Job drawing, mm, ordinate dimensions from the low corner. One solid piece. A direction names the side the tool comes from. Round coordinates to 2 decimals unless told otherwise and drop trailing zeros. Loops run counter-clockwise (first coordinate to the right, second up) from the corner with the lowest first, then second, coordinate; pieces in that order, holes last.
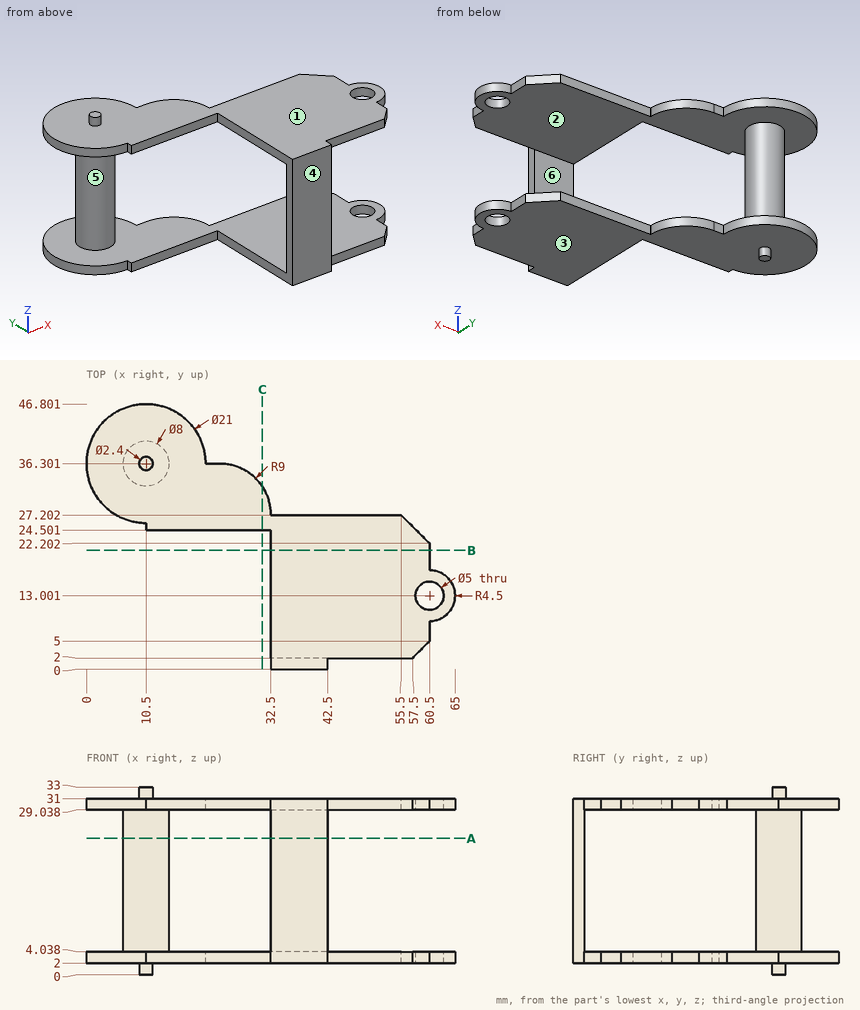
Item 1: Cut at A-A, the plane z = 24. Give the cut face in (x, y).
Answers follow:
outline: circle Ø8 at (10.5, 36.3); (32.5, 0) - (42.5, 0) - (42.5, 2) - (32.5, 2) - close
Item 2: Flat gauge pins, fed straight in: P1, Ø1.6, axis at x = 38.5, z = 3, coming from the +Y side; P2, Ø5, axis at y = 11.5, z = 28, coming from the -X side; P3, Ø2, axis at y = 21, z = 3.5, coming from the +X side; P4, Ø2, axis at x = 20, z = 26.5, coming from the +Y side. Where does each tip first touch, or does it go through?
Answers follow:
P1: stops at y = 27.2
P2: stops at x = 32.5
P3: stops at x = 60.5
P4: passes through
Item 3: Probe line 1 (Z direction, x = 51, y = 10); line 2 (Y direction, x = 35, z = 16); line 3 (Y direction, x = 11.5, z = 30.5). List the from-to ranges inside material, lowest first.
Answers follow:
line 1: z = 2 to 4.04, 29.04 to 31
line 2: y = 0 to 2
line 3: y = 24.5 to 46.75
Item 4: Two-plate mould, pull along Z, no slides. Class the marked faces 1, 2 and 3: released by +Z, released by -Z, zero draft, split by the parting line, or undercut.
Answers follow:
face 1: released by +Z
face 2: undercut
face 3: released by -Z
Item 5: 3-axis set-ups, long thin cutter, end or side, ignore diameter. For the marked faces 4, 5 and 6: which of +Z, -Z, +X, -X, +Y, -Y reach the whole face in a straight line?
Answers follow:
face 4: +Z, -Z, +X, -X, -Y
face 5: none
face 6: +X, -X, +Y
Item 6: Cut at C-C, the plane x = 31. Give the cut face in (y, z).
Answers follow:
outline: (24.5, 2) - (32.28, 2) - (32.28, 4.04) - (24.5, 4.04) - close; (24.5, 29.04) - (32.28, 29.04) - (32.28, 31) - (24.5, 31) - close
Item 7: Cut at B-B, the plane y = 21. Give the cut face in (x, z).
Answers follow:
outline: (32.5, 2) - (60.5, 2) - (60.5, 4.04) - (32.5, 4.04) - close; (32.5, 29.04) - (60.5, 29.04) - (60.5, 31) - (32.5, 31) - close
